Check sheet for the drawn part. Datum: minimum x, y, z corner. Units: mm. Give positions to 0.01 mm unless a question says otherwise; leave off trailing zeros. Order: outer loops, then holes, each group sorted by start corner. A loop starts at its lowest first (then second) coordinate and runs counter-clockwise, first axis right, second up. Notation, with made-up numbers: (9.25, 85.5) -> (45.25, 85.5) arc R28 ccw to (45.25, 104.5) -> close; hole circle Ø9 at (-36, 72). An arc over 180 degrees is marked (long way). Answer in a Markdown table with one row per item. Add a question column.
(1) Release check for a two-part mould opening along Y. For the marked faces 1, 2 and 3 record: released by +Y, released by -Y, zero draft, split by the parting line, or undercut.
(2) Cross-section at B-B (z = 15). Record the cut outline in (x, y).
(3) Go/stop test with flat-tipped pins: pin 1 (6 mm diameter, centred on x = 21.5, z = 12, fed in from +Y); pin 2 (6 mm diameter, centred on y = 17, z = 13.5, fed in from +X); pin 3 (7.5 mm diameter, centred on x = 18.5, y = 8.5, fed in from -Z). Record where each tip stops, or that it passes through.
(4) Thickness scan on L1, parallel to Y at x = 13.31, z = 7.25; L2, parallel to Y at x = 22.25, z = 6.5; L3, parallel to Z at x = 18.75, y = 21. Record the ranges inside material, lowest first. Write a range as [from, to].
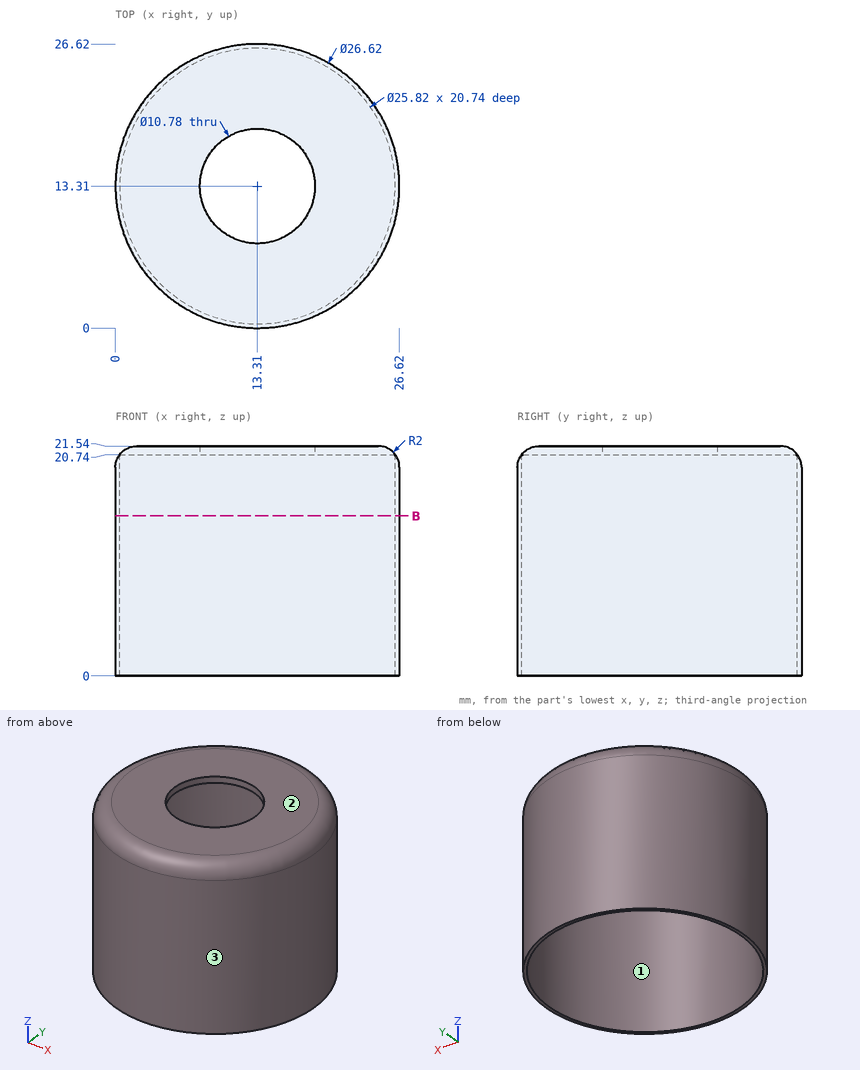
Answer below:
| question | item | result |
|---|---|---|
| 1 | face 1 | undercut |
| 1 | face 2 | zero draft |
| 1 | face 3 | split by the parting line |
| 2 | outline | circle Ø26.62 at (13.31, 13.31); hole circle Ø25.82 at (13.31, 13.31) |
| 3 | pin 1 | stops at y = 25.57 |
| 3 | pin 2 | stops at x = 26.6 |
| 3 | pin 3 | stops at z = 20.74 |
| 4 | L1 | y = [0, 0.4], [26.22, 26.62] |
| 4 | L2 | y = [3.45, 4], [22.62, 23.17] |
| 4 | L3 | z = [20.74, 21.54] |
